Design review of the part built by this model. Coordinates are the model's own, in mm. Face numbers are marked on the shaded views. A direction names the side the tool comes from. Round coordinates to 2 decimals unless told otherwise and drop trailing zeros. Order: outer loops, then holes, each group sorted by start corner. A loop starts at its lowest first (then second) coordinate and runs counter-clockwise, first axis right, second up. Notation, with made-up numbers: (11.25, 3) - (32.25, 3) arc R27 ccw to (32.25, 30) - close; hole circle Ø3 at (88.25, -33). An arc over 180 degrees is marked (long way). Use CSV: the item, a comma, the result in double quotes. Start each with the question number.
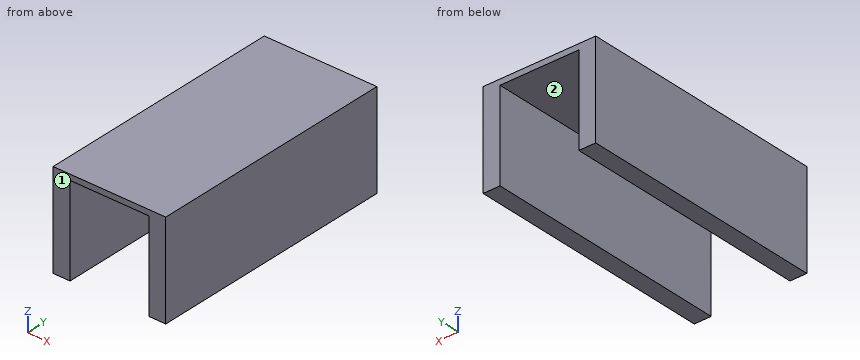
from build123d import *

# Parameters (mm, degrees)
F0_W     = 1000
F0_H     = 50
F1_DEPTH = 2200
F2_W     = 150
F2_H     = 800
F3_DEPTH = 2200


with BuildPart() as f1:
    # F0 (on Front) → F1 (new body)
    with BuildSketch(Plane.XZ):
        with Locations((-4.120639, 825)):
            Rectangle(F0_W, F0_H)
    extrude(amount=F1_DEPTH)

    # F2 (on face) → F3 (join, through all)
    with BuildSketch(Plane.XZ.offset(2200)):
        with Locations((420.879361, 400)):
            Rectangle(F2_W, F2_H)
        with Locations((-429.120639, 400)):
            Rectangle(F2_W, F2_H)
    extrude(amount=-F3_DEPTH)


solid = f1.part
Q1. Take a section at C-C (x = -228). State the section outline as (y, z) points, plus the area to 3 significant figures.
Q2. For L1, parallel to X at y = -252.5, z = 734; L2, parallel to Z at x = 202.5, y = -288, list the stretches that pass through material, from the lowest coordinate up. Write a range as [from, to].
Q3. Take a section at A-A (z = 135). State the section outline as (x, y) points.
Q4. Tool access review of the marked faces 1 and 2: name each direction out of +Z, -Z, +X, -X, +Y, -Y from which nothing blocks a thin tool from reaching the whole face with its end or side.
Q5. Take a section at B-B (y = -371). State the section outline as (x, z) points.
Q6. Clearance check with a flat-ended pin moving along its axis: pin 1 (1.5 mm diameter, centred on x = 223, y = -1852.5, fed in from -Z). State where the tip first meets the part, or that it passes through.
Findings below:
1,outline,"(-2200, 800) - (0, 800) - (0, 850) - (-2200, 850) - close"
1,area,"110,000 mm^2"
2,L1,"x = [-504.12, -354.12], [345.88, 495.88]"
2,L2,"z = [800, 850]"
3,outline,"(-504.12, -2200) - (-354.12, -2200) - (-354.12, 0) - (-504.12, 0) - close; (345.88, -2200) - (495.88, -2200) - (495.88, 0) - (345.88, 0) - close"
4,face 1,"+Z, -Z, +X, -X, -Y"
4,face 2,"-Z, +Y, -Y"
5,outline,"(-504.12, 0) - (-354.12, 0) - (-354.12, 800) - (345.88, 800) - (345.88, 0) - (495.88, 0) - (495.88, 850) - (-504.12, 850) - close"
6,pin 1,"stops at z = 800"
